```python
from build123d import *
from build123d import SkipClean  # not in build123d's __all__

# Parameters (mm, degrees)
F0_R     = 9.49325
F1_DEPTH = 35.2425
F2_R     = 19.05
F3_DEPTH = 16.0782
F4_R     = 13.335
F5_DEPTH = 28.7655
F6_R     = 3.96875
F7_DEPTH = 80.0862
F8_R     = 16.51
F8_R_2   = 9.49325
F9_DEPTH = 2.0955
F10_W    = 3.81
F10_H    = 0.508
F12_W    = 2.3495
F12_H    = 4.4069


with BuildPart() as f1:
    # F0 (on Right) → F1 (new body)
    with BuildSketch(Plane.YZ):
        Circle(F0_R)
    extrude(amount=F1_DEPTH)

    # F2 (on face) → F3 (join)
    with BuildSketch(Plane.YZ.offset(35.2425)):
        Circle(F2_R)
    extrude(amount=F3_DEPTH)

    # F4 (on face) → F5 (join)
    with BuildSketch(Plane.YZ.offset(51.3207)):
        Circle(F4_R)
    extrude(amount=F5_DEPTH)

    # F6 (on face) → F7 (cut, through all)
    with BuildSketch(Plane.YZ.offset(80.0862)):
        Circle(F6_R)
    extrude(amount=-F7_DEPTH, mode=Mode.SUBTRACT)

    # F8 (on face) → F9 (cut)
    with BuildSketch(Plane(origin=(35.2425, 0, 0), x_dir=(0, -1, 0), z_dir=(-1, 0, 0))):
        Circle(F8_R)
        Circle(F8_R_2, mode=Mode.SUBTRACT)
    with SkipClean():  # cleaning this boolean's faces spoils the solid; the shape is the same uncleaned
        extrude(amount=-F9_DEPTH, mode=Mode.SUBTRACT)

    # F10 (on Front) → F11 (revolve, cut)
    with BuildSketch(Plane.XZ):
        with Locations((36.0383225369, 9.23925)):
            Rectangle(F10_W, F10_H)
    revolve(axis=Axis((43.7559969723, 0, 0), (1, 0, 0)), mode=Mode.SUBTRACT)

    # F12 (on Front) → F13 (revolve, cut)
    with BuildSketch(Plane.XZ):
        with Locations((41.81475, 16.84655)):
            Rectangle(F12_W, F12_H)
    revolve(axis=Axis((42.9936237633, 0, 0), (1, 0, 0)), mode=Mode.SUBTRACT)

    # F14 (on Front) → F15 (revolve, cut)
    with BuildSketch(Plane.XZ):
        Polygon((6.35, 9.49325), (0, 9.49325), (0, 6.12775), align=None)
        Polygon((80.0862, 13.335), (73.7362, 13.335), (80.0862, 9.271), align=None)
    revolve(axis=Axis((41.732724756, 0, 0), (1, 0, 0)), mode=Mode.SUBTRACT)


solid = f1.part
```
Geometry check sheet. Reference: the model listing, model coordinates, mm. A direction names the side the tool comes from. Coordinates: 2 decimals unless noted, no trailing zeros. Order: outer loops, then holes, each group sorted by start corner. A loop starts at its lowest first (then second) coordinate and runs counter-clockwise, first axis right, second up. Notation, with made-up numbers: (-11.5, -38) - (29.5, -38) arc R27 cw to (29.5, 0) - close; hole circle Ø9 at (1.25, 13.5). An arc over 180 degrees is marked (long way). Answer in a Markdown table with one row per item. Add a question column.
1. Section check D-D (x = 48.5). Enter the section's corners in (y, z).
2. Section check A-A (x = 36.5). Enter the section's corners in (y, z).
3. Section check C-C (x = 59). Enter the section's corners in (y, z) (1 decimal).
4. Gauge pin test, flat ends, axial feed: pin 1 Ø1 at (x, y) = (61.5, 0) entering from +Z (3 decimals); pin 2 Ø5 at (x, y) = (50, 12) entering from -Z; pin 3 Ø8 at (y, z) = (-12, 3) entering from -X. Record the tip position at first contact, or that the pin passes through.
5. Draft check along Y on faces 1 (the face through (36.276, -15.748, 4.959)), 2 (the face through (42.99, 14, -6)), 3 (the face through (20.047, 9.055, 2.852)). Enter one of: +Y half, -Y half, draft (parallel to the pull), parting line (faces both ways), or undercut.
6. Access from +Z, -Z, +X, -X, +Y, -Y to the whole of each face (thin tool, end or side, straight path). Record for faces 4 (the face through (0, 1, -4)), 5 (the face through (35.242, -6, 16)), 6 (the face through (41.831, 14.295, -3.174)), 7 (the face through (62.372, 12.318, -5.107)), 8 (the face through (47.1, 18.17, 5.72)).
7. Section check B-B (y = 15.5). Enter the section's corners in (x, z), plus the area to 3 significant figures.
8. Material ranges on L1, parallel to Z at x = 37.7, y = 0; L2, parallel to Z at x = 36.45, y = 0; L3, parallel to X at y = 6, z = -14, recorded low to high. Write a range as [from, to].
Data:
| question | item | result |
|---|---|---|
| 1 | outline | circle Ø38.1 at (0, 0); hole circle Ø7.94 at (0, 0) |
| 2 | outline | circle Ø38.1 at (0, 0); circle Ø17.97 at (0, 0); hole circle Ø33.02 at (0, 0); hole circle Ø7.94 at (0, 0) |
| 3 | outline | circle Ø26.7 at (0, 0); hole circle Ø7.9 at (0, 0) |
| 4 | pin 1 | stops at z = 13.335 |
| 4 | pin 2 | stops at z = -16.51 |
| 4 | pin 3 | stops at x = 4.23 |
| 5 | face 1 | undercut |
| 5 | face 2 | draft |
| 5 | face 3 | parting line |
| 6 | face 4 | +Z, -Z, -X, +Y, -Y |
| 6 | face 5 | -X |
| 6 | face 6 | none |
| 6 | face 7 | +X |
| 6 | face 8 | +X, -X |
| 7 | outline | (35.24, -11.07) - (40.64, -11.07) - (40.64, 11.07) - (35.24, 11.07) - (35.24, 5.69) - (37.34, 5.69) - (37.34, -5.69) - (35.24, -5.69) - close; (42.99, -11.07) - (51.32, -11.07) - (51.32, 11.07) - (42.99, 11.07) - close |
| 7 | area | 280 mm² |
| 8 | L1 | z = [-19.05, -9.49], [-8.99, -3.97], [3.97, 8.99], [9.49, 19.05] |
| 8 | L2 | z = [-19.05, -16.51], [-8.99, -3.97], [3.97, 8.99], [16.51, 19.05] |
| 8 | L3 | x = [37.34, 40.64], [42.99, 51.32] |
